Geometry check sheet. Reference: the model listing, model coordinates, mm. A direction names the side the tool comes from. Coordinates: 2 decimals unless noted, no trailing zeros. Loops run counter-clockwise (first coordinate to the right, second up) from the corner with the lowest first, then second, coordinate; pieces in that order, holes last.
from build123d import *

# Parameters (mm, degrees)
SKETCH1_R          = 6
SKETCH2_R          = 8
CUT_EXTRUDE1_DEPTH = 10


with BuildPart() as part:
    # Sketch1 → Loft1 section 0
    with BuildSketch(Plane(origin=(0, 0, 0), x_dir=(1, 0, 0), z_dir=(0, 1, 0))):
        Circle(SKETCH1_R)
    # Sketch2 → Loft1 section 1
    with BuildSketch(Plane(origin=(0, -12, 0), x_dir=(1, 0, 0), z_dir=(0, 1, 0))):
        Circle(SKETCH2_R)
    loft()

    # Sketch4 → Cut-Extrude1 (cut)
    with BuildSketch(Plane.XZ.offset(12)):
        with BuildLine():
            ThreePointArc((3.15, 0), (-0.801366085, 3.046360517), (-2.74226184, -1.55))
            Line((-2.74226184, -1.55), (2.74226184, -1.55))
            ThreePointArc((2.74226184, -1.55), (3.046360517, -0.801366085), (3.15, 0))
        make_face()
    extrude(amount=-CUT_EXTRUDE1_DEPTH, mode=Mode.SUBTRACT)


solid = part.part
(1) Sectioned sample at B-B on y = -4.75. Record the cut outline in (x, z).
Findings:
outline: circle Ø13.58 at (0, 0); hole (-2.74, -1.55) - (2.74, -1.55) arc R3.15 ccw (long way) to start
(2) Access from +Z, -Z, +X, -X, +Y, -Y to the whole of each face (thin tool, end or side, straight path). Record for faces 4 (the flat face through (0, 0, 0)), 5 (the flat face through (0, -2, 0)).
Findings:
face 4: +Z, -Z, +X, -X, +Y
face 5: -Y
(3) Gauge pin test, flat ends, axial feed: pin 1 Ø2 at (y, z) = (-3.5, 6) entering from +X; pin 2 Ø1.5 at (y, z) = (-9.5, -4.5) entering from -X; pin 3 Ø1.4 at (x, z) = (1, -0.5) entering from -Y. Record the tip position at first contact, or that the pin passes through.
Findings:
pin 1: stops at x = 4.31
pin 2: stops at x = -6.61
pin 3: stops at y = -2
(4) Sectioned sample at A-A on x = 0. Record the cut outline in (y, z).
Findings:
outline: (-12, -8) - (0, -6) - (0, 6) - (-12, 8) - (-12, 3.15) - (-2, 3.15) - (-2, -1.55) - (-12, -1.55) - close
(5) Scan lines: L1, parallel to X at y = -6.5, z = 0; L2, parallel to Z at x = 1.25, y = -4; L3, parallel to X at y = -6, z = 2. Record each from-to range of solid material in increasing order.
Findings:
L1: x = -7.08 to -3.15, 3.15 to 7.08
L2: z = -6.55 to -1.55, 2.89 to 6.55
L3: x = -6.71 to -2.43, 2.43 to 6.71
(6) Sectioned sample at C-C on y = -1. Record the cut outline in (x, z), and give its area (3 significant figures).
Findings:
outline: circle Ø12.33 at (0, 0)
area: 119 mm2
(7) Draft check along Z on faces 1 (the conical face through (-5.39, -4.75, 4.13)), 2 (the flat face through (0, -7, -1.55)), 3 (the flat face through (0, -12, -2)). Enter one of: +Z half, -Z half, draft (parallel to the pull), parting line (faces both ways), or undercut.
Findings:
face 1: parting line
face 2: undercut
face 3: draft
(8) Sectioned sample at D-D on y = -8. Record the cut outline in (x, z).
Findings:
outline: circle Ø14.67 at (0, 0); hole (-2.74, -1.55) - (2.74, -1.55) arc R3.15 ccw (long way) to start
